The listing builds one solid part. Answer for the finished solid, in the listing's coordinates (mm). A direction names the side the tool comes from. Round coordinates to 2 decimals unless told otherwise and drop trailing zeros. Loops run counter-clockwise (first coordinate to the right, second up) from the corner with the lowest first, then second, coordinate; pieces in that order, holes last. Notation, with made-up numbers: M 41,55 L 96,55 A30 cw 96,79 Z; hole C -6,14 d10. An arc over 180 degrees is marked long. Put each result on its own line as item: value. Start each with the question number.
(1) Section B-B, the plane y = 119 is taken. Determine the outline of the cut face in (x, z), then the cut area to 3 significant figures.
(2) Section D-D, the plane y = 44.5 is taken. Determine the outline of the cut face in (x, z), then the cut area to 3 significant figures.
(3) Straight lines are drawn through the part: line 1 (Z direction, x = 0, y = 84); line 2 (Z direction, x = 0, y = 115.5); line 3 (Z direction, x = -107, y = 93). For each, find the intervals that lie inside material, in ascending order.
(4) Which of the six approach directions +Z, -Z, +X, -X, +Y, -Y give full straight-line access (tool end or side, diameter ignored) to faces 4 (the face through (-29, 115, 28)), 5 (the face through (38, 107, 15)), 6 (the face through (62, 70, -2)), 7 (the face through (100.671, 95.07, 74.643)), 8 (the face through (39, 123, 7.5))?
(5) Flat-ended cylindrical pins translate along their axes: P1, Ø10, axis at x = 90, y = 94.5, coming from the +Z side; P2, Ø12, axis at x = -37.5, z = -103, coming from the -Y side; P3, Ø1, axis at x = 29.5, z = -2, coming from the -Y side; P4, Ø8, axis at y = 88.5, z = -2, coming from the -X side. Find the tip coordinate at first contact, or state that the pin passes through.
(6) Determine the mould class of faces 1 (the face through (5.38, 80.14, -128.43)), 2 (the face through (-1.302, 95.07, -89.915)), 3 (the face through (39, 115, 11)) for opening direction X: released by +X, released by -X, zero draft, split by the parting line, or undercut.
(7) Section C-C, the plane y = 26.5 is taken. Determine the outline of the cut face in (x, z), then the cut area to 3 significant figures.
```python
from build123d import *

# Parameters (mm, degrees)
SKETCH1_R           = 30
BOSS_EXTRUDE1_DEPTH = 50
SKETCH2_R           = 60
BOSS_EXTRUDE2_DEPTH = 20
SKETCH3_R           = 150
BOSS_EXTRUDE3_DEPTH = 30
SKETCH4_R           = 50
BOSS_EXTRUDE4_DEPTH = 30
SKETCH5_R           = 15
CUT_EXTRUDE1_DEPTH  = 131
SKETCH6_R           = 20
CUT_EXTRUDE2_DEPTH  = 20
SKETCH7_R           = 10
SKETCH7_R_2         = 15
CUT_EXTRUDE3_DEPTH  = 10
SKETCH7_3_R         = 10
CUT_EXTRUDE4_DEPTH  = 101
SKETCH8_R           = 8.5
CUT_EXTRUDE6_DEPTH  = 101
SKETCH8_3_R         = 10
SKETCH8_3_R_2       = 8.5
CUT_EXTRUDE7_DEPTH  = 10
SKETCH10_W          = 32.181548772
SKETCH10_H          = 15
CUT_EXTRUDE8_DEPTH  = 30
SKETCH11_W          = 24.632188436
SKETCH11_H          = 30
CUT_EXTRUDE9_DEPTH  = 15
CUT_EXTRUDE10_DEPTH = 40
FILLET1_R           = 5


with BuildPart() as part:
    # Sketch1 → Boss-Extrude1 (new body)
    with BuildSketch(Plane(origin=(0, 0, 0), x_dir=(1, 0, 0), z_dir=(0, 1, 0))):
        Circle(SKETCH1_R)
    extrude(amount=BOSS_EXTRUDE1_DEPTH)

    # Sketch2 → Boss-Extrude2 (add)
    with BuildSketch(Plane(origin=(0, 50, 0), x_dir=(1, 0, 0), z_dir=(0, 1, 0))):
        Circle(SKETCH2_R)
    extrude(amount=BOSS_EXTRUDE2_DEPTH)

    # Sketch3 → Boss-Extrude3 (add)
    with BuildSketch(Plane(origin=(0, 70, 0), x_dir=(1, 0, 0), z_dir=(0, 1, 0))):
        Circle(SKETCH3_R)
    extrude(amount=BOSS_EXTRUDE3_DEPTH)

    # Sketch4 → Boss-Extrude4 (add)
    with BuildSketch(Plane(origin=(0, 100, 0), x_dir=(1, 0, 0), z_dir=(0, 1, 0))):
        Circle(SKETCH4_R)
    extrude(amount=BOSS_EXTRUDE4_DEPTH)

    # Sketch5 → Cut-Extrude1 (cut, through all)
    with BuildSketch(Plane(origin=(0, 130, 0), x_dir=(1, 0, 0), z_dir=(0, 1, 0))):
        Circle(SKETCH5_R)
    extrude(amount=-CUT_EXTRUDE1_DEPTH, mode=Mode.SUBTRACT)

    # Sketch6 → Cut-Extrude2 (cut)
    with BuildSketch(Plane(origin=(0, 130, 0), x_dir=(1, 0, 0), z_dir=(0, 1, 0))):
        Circle(SKETCH6_R)
    extrude(amount=-CUT_EXTRUDE2_DEPTH, mode=Mode.SUBTRACT)

    # Sketch7 → Cut-Extrude3 (cut)
    with BuildSketch(Plane(origin=(0, 100, 0), x_dir=(1, 0, 0), z_dir=(0, 1, 0))):
        with Locations((-103.923048454, -60)):
            Circle(SKETCH7_R)
        with Locations((-103.923048454, -60)):
            Circle(SKETCH7_R_2)
        with Locations((-103.923048454, -60)):
            Circle(SKETCH7_R, mode=Mode.SUBTRACT)
        with Locations((-103.923048454, 60)):
            Circle(SKETCH7_R)
        with Locations((-103.923048454, 60)):
            Circle(SKETCH7_R_2)
        with Locations((-103.923048454, 60)):
            Circle(SKETCH7_R, mode=Mode.SUBTRACT)
        with Locations((0, 120)):
            Circle(SKETCH7_R)
        with Locations((0, 120)):
            Circle(SKETCH7_R_2)
        with Locations((0, 120)):
            Circle(SKETCH7_R, mode=Mode.SUBTRACT)
        with Locations((103.923048454, 60)):
            Circle(SKETCH7_R_2)
        with Locations((103.923048454, 60)):
            Circle(SKETCH7_R, mode=Mode.SUBTRACT)
        with Locations((103.923048454, 60)):
            Circle(SKETCH7_R)
        with Locations((103.923048454, -60)):
            Circle(SKETCH7_R_2)
        with Locations((103.923048454, -60)):
            Circle(SKETCH7_R, mode=Mode.SUBTRACT)
        with Locations((103.923048454, -60)):
            Circle(SKETCH7_R)
        with Locations((0, -120)):
            Circle(SKETCH7_R_2)
        with Locations((0, -120)):
            Circle(SKETCH7_R, mode=Mode.SUBTRACT)
        with Locations((0, -120)):
            Circle(SKETCH7_R)
    extrude(amount=-CUT_EXTRUDE3_DEPTH, mode=Mode.SUBTRACT)

    # Sketch7<3> → Cut-Extrude4 (cut, through all)
    with BuildSketch(Plane(origin=(0, 100, 0), x_dir=(1, 0, 0), z_dir=(0, 1, 0))):
        with Locations((-103.923048454, -60)):
            Circle(SKETCH7_3_R)
        with Locations((-103.923048454, 60)):
            Circle(SKETCH7_3_R)
        with Locations((0, 120)):
            Circle(SKETCH7_3_R)
        with Locations((103.923048454, 60)):
            Circle(SKETCH7_3_R)
        with Locations((103.923048454, -60)):
            Circle(SKETCH7_3_R)
        with Locations((0, -120)):
            Circle(SKETCH7_3_R)
    extrude(amount=-CUT_EXTRUDE4_DEPTH, mode=Mode.SUBTRACT)

    # Sketch8 → Cut-Extrude6 (cut, through all)
    with BuildSketch(Plane(origin=(0, 100, 0), x_dir=(1, 0, 0), z_dir=(0, 1, 0))):
        with Locations((0, -80)):
            Circle(SKETCH8_R)
        with Locations((0, 80)):
            Circle(SKETCH8_R)
    extrude(amount=-CUT_EXTRUDE6_DEPTH, mode=Mode.SUBTRACT)

    # Sketch8<3> → Cut-Extrude7 (cut)
    with BuildSketch(Plane(origin=(0, 100, 0), x_dir=(1, 0, 0), z_dir=(0, 1, 0))):
        with Locations((0, -80)):
            Circle(SKETCH8_3_R)
        with Locations((0, -80)):
            Circle(SKETCH8_3_R_2, mode=Mode.SUBTRACT)
        with Locations((0, 80)):
            Circle(SKETCH8_3_R)
        with Locations((0, 80)):
            Circle(SKETCH8_3_R_2, mode=Mode.SUBTRACT)
    extrude(amount=-CUT_EXTRUDE7_DEPTH, mode=Mode.SUBTRACT)

    # Sketch10 → Cut-Extrude8 (cut)
    with BuildSketch(Plane(origin=(0, 130, 0), x_dir=(1, 0, 0), z_dir=(0, 1, 0))):
        Polygon((-20.949803335, -21.286123785), (-7.959422279, -28.786123785), (-24.050196665, -56.656162555), (-37.040577721, -49.156162555), align=None)
        with Locations((45, 0)):
            Rectangle(SKETCH10_W, SKETCH10_H)
        Polygon((-7.959422279, 28.786123785), (-20.949803335, 21.286123785), (-37.040577721, 49.156162555), (-24.050196665, 56.656162555), align=None)
    extrude(amount=-CUT_EXTRUDE8_DEPTH, mode=Mode.SUBTRACT)

    # Sketch11 → Cut-Extrude9 (cut)
    with BuildSketch(Plane(origin=(0, 100, 0), x_dir=(1, 0, 0), z_dir=(0, 1, 0))):
        with Locations((41.225319832, 0)):
            Rectangle(SKETCH11_W, SKETCH11_H)
        Polygon((-27.444993864, -17.536123785), (-1.46423175, -32.536123785), (-13.780325968, -53.868224722), (-39.761088082, -38.868224722), align=None)
        Polygon((-1.46423175, 32.536123785), (-27.444993864, 17.536123785), (-39.761088082, 38.868224722), (-13.780325968, 53.868224722), align=None)
    extrude(amount=CUT_EXTRUDE9_DEPTH, mode=Mode.SUBTRACT)

    # Sketch12 → Cut-Extrude10 (cut)
    with BuildSketch(Plane.XZ):
        with BuildLine():
            Line((-28.75, -8.569568251), (-28.75, 8.569568251))
            ThreePointArc((-28.75, 8.569568251), (-30, 0), (-28.75, -8.569568251))
        make_face()
        with BuildLine():
            ThreePointArc((30, 0), (29.685855218, 4.330127019), (28.75, 8.569568251))
            Line((28.75, 8.569568251), (28.75, -8.569568251))
            ThreePointArc((28.75, -8.569568251), (29.685855218, -4.330127019), (30, 0))
        make_face()
    extrude(amount=-CUT_EXTRUDE10_DEPTH, mode=Mode.SUBTRACT)

    # Fillet1
    fillet1_edges = [part.edges().sort_by_distance(p)[0] for p in [
        (-150, 70, 0),
        (-150, 100, 0),
    ]]
    fillet(fillet1_edges, radius=FILLET1_R)


solid = part.part
```
Recorded:
1. outline: M -31.21,-39.06 L -20.95,-21.29 L -7.96,-28.79 L -18.22,-46.56 A50 ccw 49.43,-7.5 L 28.91,-7.5 L 28.91,7.5 L 49.43,7.5 A50 ccw -18.22,46.56 L -7.96,28.79 L -20.95,21.29 L -31.21,39.06 A50 ccw Z; hole C 0,0 d40
1. area: 5,660 mm²
2. outline: C 0,0 d60; hole C 0,0 d30
2. area: 2,120 mm²
3. line 1: z = -150 to -130, -110 to -88.5, -71.5 to -15, 15 to 71.5, 88.5 to 110, 130 to 150
3. line 2: z = -50 to -20, 20 to 50
3. line 3: z = -105.12 to -74.68, -45.32 to 45.32, 74.68 to 105.12
4. face 4: +Z
4. face 5: +X
4. face 6: -Y
4. face 7: +Y
4. face 8: +X, +Y
5. P1: stops at z = 123.59
5. P2: stops at y = 70
5. P3: stops at y = 40
5. P4: stops at x = -150
6. face 1: undercut
6. face 2: undercut
6. face 3: zero draft
7. outline: M -28.75,-8.57 A30 ccw 28.75,-8.57 L 28.75,8.57 A30 ccw -28.75,8.57 Z; hole C 0,0 d30
7. area: 2,090 mm²
